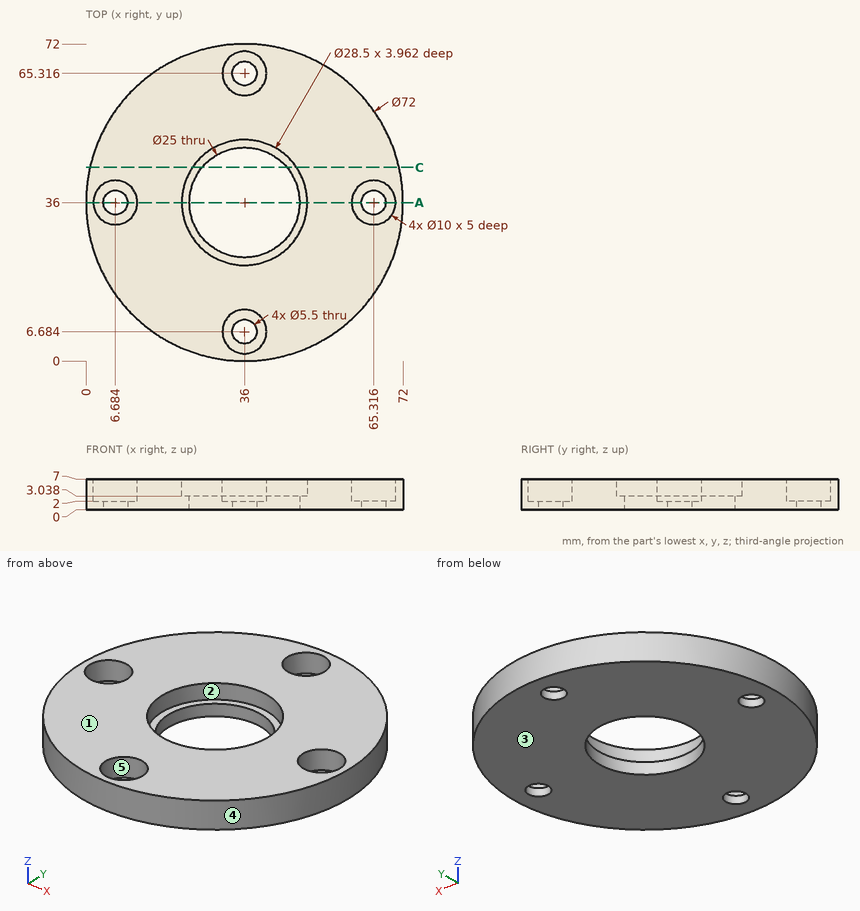
Geometry: see drawing. Coordinates: mm, zero at the bounding-box minimum. A direction names the side the tool comes from. Coordinates: 2 decimals unless noted, no trailing zeros. Loops run counter-clockwise (first coordinate to the right, second up) from the corner with the lowest first, then second, coordinate; pieces in that order, holes last. Notation, with made-up numbers: (37.5, -29.5) - (60.5, -29.5) arc R31 ccw to (60.5, 8.5) - close; hole circle Ø9 at (60, 31). An arc over 180 degrees is marked (long way). Answer as CSV lines item,"result".
1. Contact query for flat-ended pins moving along their axis: pin 1 (1.5 mm diameter, centred on y = 17, z = 4.5, fed in from +X); pin 2 (5 mm diameter, centred on x = 66.5, y = 35, fed in from +Z); pin 3 (23 mm diameter, centred on x = 36, y = 36, fed in from +Z); pin 4 (1.5 mm diameter, centred on x = 46, z = 2.5, fed in from +Y). Output: stop coordinate, or through.
Established:
pin 1,"stops at x = 67.03"
pin 2,"stops at z = 2"
pin 3,"passes through"
pin 4,"stops at y = 70.79"
2. Mould query, pull axis X, two halves, no side actions, for the marked faces 3, 4 and 5. Classes: released by +X, released by -X, zero draft, split by the parting line, or undercut.
Established:
face 3,"zero draft"
face 4,"split by the parting line"
face 5,"undercut"
3. Section C-C (y = 44). Return loops of the section in (x, z) (1 decimal).
Established:
outline,"(0.9, 0) - (26.4, 0) - (26.4, 3) - (24.2, 3) - (24.2, 7) - (0.9, 7) - close; (45.6, 0) - (71.1, 0) - (71.1, 7) - (47.8, 7) - (47.8, 3) - (45.6, 3) - close"
4. Section A-A (y = 36). Count the separate pieces of the cut face and the enclosed holes in it, then the cut area to 3 significant figures.
Established:
separate pieces,"4"
enclosed holes,"0"
area,"193 mm2"
5. Ray query, line 1 (Y direction, x = 36, z = 1.1) (1 decimal); line 2 (Y direction, x = 62.5, z = 6.75) (1 decimal); line 3 (X direction, y = 29.5, z = 4.5). Return the intervals inside material, ascending.
Established:
line 1,"y = 0 to 3.9, 9.4 to 23.5, 48.5 to 62.6, 68.1 to 72"
line 2,"y = 11.6 to 31.9, 40.1 to 60.4"
line 3,"x = 0.59 to 23.32, 48.68 to 71.41"
6. Reachability of the marked faces 1 and 2 from +Z, -Z, +X, -X, +Y, -Y: full face, straight path, thin tool, end or side. Return the list, or none.
Established:
face 1,"+Z, +X, -X, +Y, -Y"
face 2,"+Z"
